from build123d import *

# Parameters (mm, degrees)
F0_W     = 16
F0_H     = 8
F1_DEPTH = 3
F2_R     = 2.5
F3_DEPTH = 2
F4_W     = 14
F4_H     = 6
F5_DEPTH = 2
F6_R     = 1.5
F6_R_2   = 0.75
F7_DEPTH = 2
F8_R     = 1
F9_DEPTH = 1


with BuildPart() as f1:
    # F0 (on Top) → F1 (new body)
    with BuildSketch(Plane.XY):
        with Locations((17.171192, -5.046524)):
            Rectangle(F0_W, F0_H)
    extrude(amount=F1_DEPTH)

    # F2 (on face) → F3 (join)
    with BuildSketch(Plane.XY.offset(3)):
        with Locations((13.171192, -5.046524)):
            Circle(F2_R)
        with Locations((21.171192, -5.046524)):
            Circle(F2_R)
    extrude(amount=F3_DEPTH)

    # F4 (on face) → F5 (cut)
    with BuildSketch(Plane(origin=(0, 0, 0), x_dir=(1, 0, 0), z_dir=(0, 0, -1))):
        with Locations((17.171192, 5.18152)):
            Rectangle(F4_W, F4_H)
    extrude(amount=-F5_DEPTH, mode=Mode.SUBTRACT)

    # F6 (on face) → F7 (join)
    with BuildSketch(Plane(origin=(0, 0, 2), x_dir=(1, 0, 0), z_dir=(0, 0, -1))):
        with Locations((17.171192, 5.18152)):
            Circle(F6_R)
        with Locations((17.171192, 5.18152)):
            Circle(F6_R_2, mode=Mode.SUBTRACT)
    extrude(amount=F7_DEPTH)

    # F8 (on face) → F9 (cut)
    with BuildSketch(Plane(origin=(0, 0, 2), x_dir=(1, 0, 0), z_dir=(0, 0, -1))):
        with Locations((12.171192, 5.18152)):
            Circle(F8_R)
        with Locations((22.171192, 5.18152)):
            Circle(F8_R)
    extrude(amount=-F9_DEPTH, mode=Mode.SUBTRACT)


solid = f1.part
Source: CAD feature listing. Evaluate the final solid. Frame: model axes, mm. A direction names the side the tool comes from. Round coordinates to 2 decimals unless told otherwise and drop trailing zeros. Loops run counter-clockwise (first coordinate to the right, second up) from the corner with the lowest first, then second, coordinate; pieces in that order, holes last. Notation, with made-up numbers: (24.25, 2.5) - (36.25, 2.5) arc R27 ccw to (36.25, 39.5) - close; hole circle Ø8 at (24, -11). An arc over 180 degrees is marked (long way). Write item = value, one per line. Start each with the question number.
(1) Pin query (flat end, axial travel): pin 1 (1.5 mm diameter, centred on x = 16, y = -7, fed in from +Z); pin 2 (3 mm diameter, centred on x = 16, y = -7, fed in from +Z); pin 3 (1.5 mm diameter, centred on y = -6.5, z = 4, fed in from -X); pin 4 (2 mm diameter, centred on x = 12, y = -5.5, fed in from -Z). Return the tip coordinate at first contact, or that it passes through.
(2) Section query C-C, the plane y = -2. Output: boundary loops of the cut face in (x, z).
(3) Pull-direction query (Y, two-part tool) for faces 4 (the face through (17, -9.047, 1)), 5 (the face through (16.576, -4.725, 1.014)), 6 (the face through (21, -5, 5)); classes: +Y half, -Y half, draft (parallel to the pull), parting line (faces both ways), or undercut.
(4) Section query A-A, the plane z = 1.75. Output: boundary loops of the cut face in (x, y), plus the area to 3 significant figures.
(5) Ray query, line 1 along Y through (x, z) = (24, 1.75); line 2 along X through (y, z) = (-5.25, 1.3); line 3 along X through (y, z) = (-8, 1.95). Return the intervals inside material, ascending. Write a range as from..to.
(6) Section query D-D, the plane z = 3.95. Output: boundary loops of the cut face in (x, y).
(7) Set-up query: faces 1 (the face through (17, -8.182, 1)), 2 (the face through (19.19, -6.57, 3.99)), 3 (the face through (9.171, -5, 1)). Return all of +Z, -Z, +X, -X, +Y, -Y with unobstructed straight access to the full face (end or side cutting, diameter ignored); none if empty.
(8) Section query B-B, the plane x = 19.25. Output: boundary loops of the cut face in (y, z), plus the area to 3 significant figures.
Conclusion:
q1.pin_1 = 3
q1.pin_2 = 5
q1.pin_3 = 10.77
q1.pin_4 = 2
q2.outline = (9.17, 0) - (25.17, 0) - (25.17, 3) - (9.17, 3) - close
q3.face_4 = -Y half
q3.face_5 = undercut
q3.face_6 = draft
q4.outline = (9.17, -9.05) - (25.17, -9.05) - (25.17, -1.05) - (9.17, -1.05) - close; circle Ø3 at (17.17, -5.18); hole (10.17, -8.18) - (24.17, -8.18) - (24.17, -2.18) - (10.17, -2.18) - close; hole circle Ø1.5 at (17.17, -5.18)
q4.area = 49.3 mm2
q5.line_1 = -9.05..-8.18, -2.18..-1.05
q5.line_2 = 9.17..10.17, 15.67..16.42, 17.92..18.67, 24.17..25.17
q5.line_3 = 9.17..10.17, 24.17..25.17
q6.outline = circle Ø5 at (13.17, -5.05); circle Ø5 at (21.17, -5.05)
q7.face_1 = -Z
q7.face_2 = +Z
q7.face_3 = +Z, -Z, -X, +Y, -Y
q8.outline = (-9.05, 0) - (-8.18, 0) - (-8.18, 2) - (-2.18, 2) - (-2.18, 0) - (-1.05, 0) - (-1.05, 3) - (-3.45, 3) - (-3.45, 5) - (-6.65, 5) - (-6.65, 3) - (-9.05, 3) - close
q8.area = 18.4 mm2
